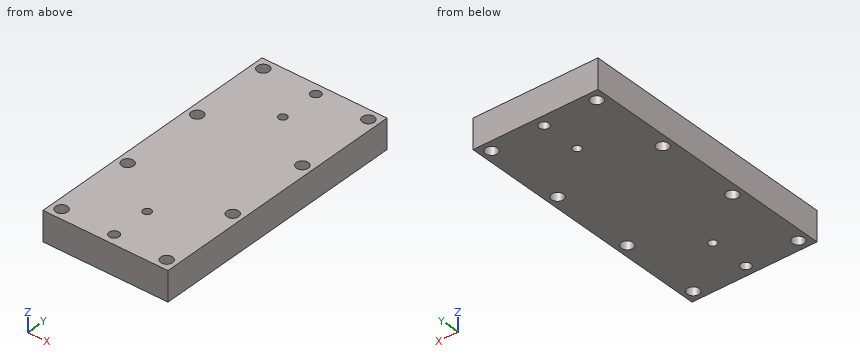
```python
from build123d import *

# Parameters (mm, degrees)
SKETCH1_W           = 63
SKETCH1_H           = 132.7
SKETCH1_R           = 3
BOSS_EXTRUDE1_DEPTH = 15
SETSCREWS_D         = 4.2
SCREWHOLES_D        = 5


with BuildPart() as part:
    # Sketch1 → Boss-Extrude1 (new body)
    with BuildSketch(Plane.XY):
        with Locations((0, 41.1)):
            Rectangle(SKETCH1_W, SKETCH1_H)
        with Locations((-26.5, 20)):
            Circle(SKETCH1_R, mode=Mode.SUBTRACT)
        with Locations((-26.5, -20)):
            Circle(SKETCH1_R, mode=Mode.SUBTRACT)
        with Locations((26.5, -20)):
            Circle(SKETCH1_R, mode=Mode.SUBTRACT)
        with Locations((26.5, 20)):
            Circle(SKETCH1_R, mode=Mode.SUBTRACT)
        with Locations((-26.5, 102.2)):
            Circle(SKETCH1_R, mode=Mode.SUBTRACT)
        with Locations((-26.5, 62.2)):
            Circle(SKETCH1_R, mode=Mode.SUBTRACT)
        with Locations((26.5, 62.2)):
            Circle(SKETCH1_R, mode=Mode.SUBTRACT)
        with Locations((26.5, 102.2)):
            Circle(SKETCH1_R, mode=Mode.SUBTRACT)
    extrude(amount=BOSS_EXTRUDE1_DEPTH)

    # setscrews (through all)
    with Locations(Plane(origin=(0, 82.2, 15), x_dir=(1, 0, 0), z_dir=(0, 0, 1))):
        with Locations((0, 0), (0, -82.2)):
            Hole(SETSCREWS_D / 2)

    # screwHoles (through all)
    with Locations(Plane(origin=(0, 102.2, 15), x_dir=(1, 0, 0), z_dir=(0, 0, 1))):
        with Locations((0, 0), (0, -122.2)):
            Hole(SCREWHOLES_D / 2)


solid = part.part
```
Model file for the job. Use its own axes, mm. Coordinates: 2 decimals unless noted, no trailing zeros. Write each loop counter-clockwise with the first axis right and the second up, starting at its lowest first coordinate (ties: lowest second). Pieces come first, ordered by that corner, then holes. Notation, with made-up numbers: (-16, 84) - (-9, 84) arc R12 cw to (-9, 100) - close; hole circle Ø5 at (-13, -23). An arc over 180 degrees is marked (long way). One line per item, written item: value. Start each with the question number.
1. Flat gauge pin, fed straight in: pin 1 (3.5 mm diameter, centred on x = 26.5, y = 62.2, fed in from -Z). Where does the tip first touch, or does it go through?
2. Slice it at C-C (x = 0). Write the cut outline in (y, z), plus the area to 3 significant figures.
3. Slice it at B-B (z = 1.75). Count the separate pieces of the cut face and the enclosed holes in it, plus the area to 3 significant figures.
4. Probe line 1 (Y direction, x = -26.5, z = 4.5); line 2 (X direction, y = 102, z = 10.5); line 3 (Y direction, x = -24, z = 14.5). List the from-to ranges inside material, lowest first. Write a range as from..to.
5. Slice it at D-D (y = -20). Write the cut outline in (x, z).
6. Slice it at A-A (y = 20). Write the cut outline in (x, z).
Answers below:
1. pin 1: passes through
2. outline: (-25.25, 0) - (-22.5, 0) - (-22.5, 15) - (-25.25, 15) - close; (-17.5, 0) - (-2.1, 0) - (-2.1, 15) - (-17.5, 15) - close; (2.1, 0) - (80.1, 0) - (80.1, 15) - (2.1, 15) - close; (84.3, 0) - (99.7, 0) - (99.7, 15) - (84.3, 15) - close; (104.7, 0) - (107.45, 0) - (107.45, 15) - (104.7, 15) - close
2. area: 1,710 mm^2
3. separate pieces: 1
3. enclosed holes: 12
3. area: 8,070 mm^2
4. line 1: y = -25.25..-23, -17..17, 23..59.2, 65.2..99.2, 105.2..107.45
4. line 2: x = -31.5..-29.49, -23.51..-2.49, 2.49..23.51, 29.49..31.5
4. line 3: y = -25.25..-21.66, -18.34..18.34, 21.66..60.54, 63.86..100.54, 103.86..107.45
5. outline: (-31.5, 0) - (-29.5, 0) - (-29.5, 15) - (-31.5, 15) - close; (-23.5, 0) - (-2.5, 0) - (-2.5, 15) - (-23.5, 15) - close; (2.5, 0) - (23.5, 0) - (23.5, 15) - (2.5, 15) - close; (29.5, 0) - (31.5, 0) - (31.5, 15) - (29.5, 15) - close
6. outline: (-31.5, 0) - (-29.5, 0) - (-29.5, 15) - (-31.5, 15) - close; (-23.5, 0) - (23.5, 0) - (23.5, 15) - (-23.5, 15) - close; (29.5, 0) - (31.5, 0) - (31.5, 15) - (29.5, 15) - close
